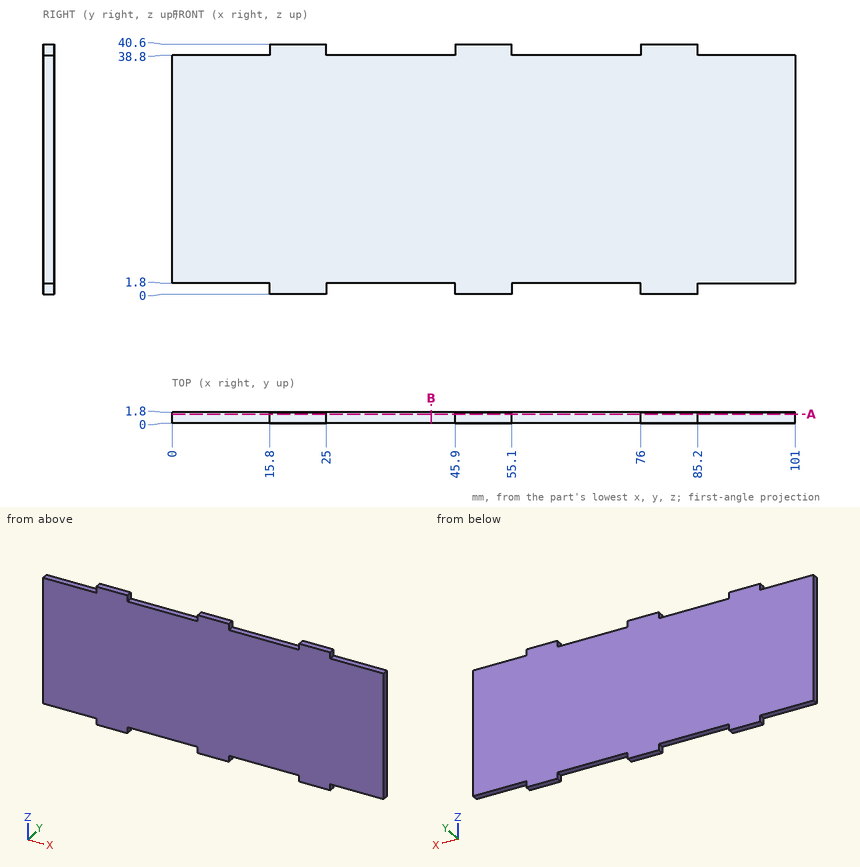
Geometry check sheet. Reference: drawing and pictorial views, mm from the part's lowest x, y, z. Give positions to 0.01 mm unless a question says otherwise; leave off trailing zeros. Order: outer loops, then holes, each group sorted by start corner. A loop starts at its lowest first (then second) coordinate and runs counter-clockwise, first axis right, second up. Notation, with made-up numbers: M -37,41.25 L -5,41.25 A24 ccw -5,76.25 Z; hole C 77.5,58.25 d2. An arc over 180 degrees is marked long. Return JSON: item names as keys, results as strings. Group by question number.
1) Go/stop test with flat-tipped pins: pin 1 Ø0.5 at (y, z) = (0.5, 1) entering from -X; pin 2 Ø0.9 at (y, z) = (1, 0.5) entering from +X; pin 3 Ø0.5 at (x, y) = (66.5, 1.5) entering from +Z. Record where each tip stops, or that it passes through.
2) Scan lines: line 1 (X direction, y = 0.5, z = 39); line 2 (Z direction, x = 88.5, y = 1.2). Record each from-to range of solid material in increasing order.
3) Section check A-A on y = 1.5. Record the cut outline in (x, z), and give its area (3 significant figures).
4) Section check B-B on x = 42. Record the cut outline in (y, z), and give its area (3 significant figures).
Answer block:
{
 "1": {"pin 1": "stops at x = 15.8", "pin 2": "stops at x = 85.2", "pin 3": "stops at z = 38.8"},
 "2": {"line 1": "x = 15.8 to 25, 45.9 to 55.1, 76 to 85.2", "line 2": "z = 1.8 to 38.8"},
 "3": {"outline": "M 0,1.8 L 15.8,1.8 L 15.8,0 L 25,0 L 25,1.8 L 45.9,1.8 L 45.9,0 L 55.1,0 L 55.1,1.8 L 76,1.8 L 76,0 L 85.2,0 L 85.2,1.8 L 101,1.8 L 101,38.8 L 85.2,38.8 L 85.2,40.6 L 76,40.6 L 76,38.8 L 55.1,38.8 L 55.1,40.6 L 45.9,40.6 L 45.9,38.8 L 25,38.8 L 25,40.6 L 15.8,40.6 L 15.8,38.8 L 0,38.8 Z", "area": "3,840 mm^2"},
 "4": {"outline": "M 0,1.8 L 1.8,1.8 L 1.8,38.8 L 0,38.8 Z", "area": "66.6 mm^2"}
}
